```python
from build123d import *

# Parameters (mm, degrees)
SKETCH1_W                      = 133.5
SKETCH1_H                      = 34
BOSS_EXTRUDE1_DEPTH            = 1
SKETCH2_W                      = 10
SKETCH2_H                      = 8.625
BOSS_EXTRUDE2_DEPTH            = 15
SKETCH2_3_W                    = 10
SKETCH2_3_H                    = 16.75
BOSS_EXTRUDE3_DEPTH            = 6.5
CBORE_FOR_M3_SHCS1_D           = 3.4
CBORE_FOR_M3_SHCS1_CBORE_D     = 6.5
CBORE_FOR_M3_SHCS1_CBORE_DEPTH = 3
CHAMFER1_SIZE                  = 0.5
CHAMFER2_SIZE                  = 0.5
CUT_EXTRUDE1_DEPTH             = 71.495123945
LPATTERN1_COUNT                = 3
LPATTERN1_PITCH                = 18.475
MIRROR2_COPY_1_DEPTH           = 71.495123945
MIRROR2_COPY_2_DEPTH           = 71.495123945
MIRROR2_COPY_3_DEPTH           = 71.495123945
CHAMFER3_SIZE                  = 1
INTERSECT1_START               = 14
INTERSECT1_OUTLINE_R           = 1.7
INTERSECT1_DEPTH               = 1


# Read off the part's stored shape, not the designer's step: Intersect1
with BuildPart() as part:
    # Sketch1 → Boss-Extrude1 (new body)
    with BuildSketch(Plane.XY):
        Rectangle(SKETCH1_W, SKETCH1_H)
    extrude(amount=BOSS_EXTRUDE1_DEPTH)

    # Sketch2 → Boss-Extrude2 (add)
    with BuildSketch(Plane.XY):
        with Locations((61.75, -12.6875)):
            Rectangle(SKETCH2_W, SKETCH2_H)
        with Locations((61.75, 12.6875)):
            Rectangle(SKETCH2_W, SKETCH2_H)
    boss_extrude2 = extrude(amount=BOSS_EXTRUDE2_DEPTH)

    # Sketch2<3> → Boss-Extrude3 (add)
    with BuildSketch(Plane.XY):
        with Locations((61.75, 0)):
            Rectangle(SKETCH2_3_W, SKETCH2_3_H)
    boss_extrude3 = extrude(amount=BOSS_EXTRUDE3_DEPTH)

    # CBORE for M3 SHCS1 (through all)
    with Locations(Plane(origin=(0, 0, 0), x_dir=(-1, 0, 0), z_dir=(0, 0, -1))):
        with Locations((-61.75, 12.75), (-61.75, -12.75)):
            cbore_for_m3_shcs1 = CounterBoreHole(CBORE_FOR_M3_SHCS1_D / 2, CBORE_FOR_M3_SHCS1_CBORE_D / 2, CBORE_FOR_M3_SHCS1_CBORE_DEPTH)

    # Chamfer1
    chamfer1_edges = [part.edges().sort_by_distance(p)[0] for p in [
        (61.75, 8.375, 6.5),
        (61.75, -8.375, 6.5),
    ]]
    chamfer(chamfer1_edges, length=CHAMFER1_SIZE)

    # Mirror1: Boss-Extrude2, Boss-Extrude3, CBORE for M3 SHCS1 across plane
    add(boss_extrude2.mirror(Plane(origin=(0, 0, 0), x_dir=(0, 0, 1), z_dir=(1, 0, 0))))
    add(boss_extrude3.mirror(Plane(origin=(0, 0, 0), x_dir=(0, 0, 1), z_dir=(1, 0, 0))))
    add(cbore_for_m3_shcs1.mirror(Plane(origin=(0, 0, 0), x_dir=(0, 0, 1), z_dir=(1, 0, 0))), mode=Mode.SUBTRACT)

    # Chamfer2
    chamfer2_edges = [part.edges().sort_by_distance(p)[0] for p in [
        (-65, -12.75, 0),
        (-65, 12.75, 0),
        (65, -12.75, 0),
        (65, 12.75, 0),
    ]]
    chamfer(chamfer2_edges, length=CHAMFER2_SIZE)

    # Sketch6 → Cut-Extrude1 (cut, through all)
    with BuildSketch(Plane.XY):
        Polygon((-7.505553499, 15), (0, 2), (7.505553499, 15), align=None)
        Polygon((-16.743157806, 1), (-1.732050808, 1), (-9.237604307, 14), align=None)
        Polygon((-16.743157806, -1), (-9.237604307, -14), (-1.732050808, -1), align=None)
        Polygon((1.732050808, 1), (16.743157806, 1), (9.237604307, 14), align=None)
        Polygon((1.732050808, -1), (9.237604307, -14), (16.743157806, -1), align=None)
        Polygon((-7.505553499, -15), (7.505553499, -15), (0, -2), align=None)
    cut_extrude1 = extrude(amount=CUT_EXTRUDE1_DEPTH, mode=Mode.SUBTRACT)

    # LPattern1: Cut-Extrude1 ×3
    with Locations(*[(-i * LPATTERN1_PITCH, 0, 0) for i in range(1, LPATTERN1_COUNT)]):
        add(cut_extrude1, mode=Mode.SUBTRACT)

    # Mirror2 copy 1 sketch → Mirror2 copy 1 (cut, through all)
    with BuildSketch(Plane(origin=(18.475, 0, 0), x_dir=(-1, 0, 0), z_dir=(0, 0, 1))):
        Polygon((-7.505553499, -15), (0, -2), (7.505553499, -15), align=None)
        Polygon((-16.743157806, -1), (-1.732050808, -1), (-9.237604307, -14), align=None)
        Polygon((-16.743157806, 1), (-9.237604307, 14), (-1.732050808, 1), align=None)
        Polygon((1.732050808, -1), (16.743157806, -1), (9.237604307, -14), align=None)
        Polygon((1.732050808, 1), (9.237604307, 14), (16.743157806, 1), align=None)
        Polygon((-7.505553499, 15), (7.505553499, 15), (0, 2), align=None)
    extrude(amount=MIRROR2_COPY_1_DEPTH, mode=Mode.SUBTRACT)

    # Mirror2 copy 2 sketch → Mirror2 copy 2 (cut, through all)
    with BuildSketch(Plane(origin=(36.95, 0, 0), x_dir=(-1, 0, 0), z_dir=(0, 0, 1))):
        Polygon((-7.505553499, -15), (0, -2), (7.505553499, -15), align=None)
        Polygon((-16.743157806, -1), (-1.732050808, -1), (-9.237604307, -14), align=None)
        Polygon((-16.743157806, 1), (-9.237604307, 14), (-1.732050808, 1), align=None)
        Polygon((1.732050808, -1), (16.743157806, -1), (9.237604307, -14), align=None)
        Polygon((1.732050808, 1), (9.237604307, 14), (16.743157806, 1), align=None)
        Polygon((-7.505553499, 15), (7.505553499, 15), (0, 2), align=None)
    extrude(amount=MIRROR2_COPY_2_DEPTH, mode=Mode.SUBTRACT)

    # Mirror2 copy 3 sketch → Mirror2 copy 3 (cut, through all)
    with BuildSketch(Plane(origin=(0, 0, 0), x_dir=(-1, 0, 0), z_dir=(0, 0, 1))):
        Polygon((-7.505553499, -15), (0, -2), (7.505553499, -15), align=None)
        Polygon((-16.743157806, -1), (-1.732050808, -1), (-9.237604307, -14), align=None)
        Polygon((-16.743157806, 1), (-9.237604307, 14), (-1.732050808, 1), align=None)
        Polygon((1.732050808, -1), (16.743157806, -1), (9.237604307, -14), align=None)
        Polygon((1.732050808, 1), (9.237604307, 14), (16.743157806, 1), align=None)
        Polygon((-7.505553499, 15), (7.505553499, 15), (0, 2), align=None)
    extrude(amount=MIRROR2_COPY_3_DEPTH, mode=Mode.SUBTRACT)

    # Chamfer3
    chamfer3_edges = [part.edges().sort_by_distance(p)[0] for p in [
        (66.75, -17, 7.5),
        (-66.75, -17, 7.5),
        (-66.75, 17, 7.5),
        (66.75, 17, 7.5),
    ]]
    chamfer(chamfer3_edges, length=CHAMFER3_SIZE)

    # Intersect1 outline → Intersect1 (cut)
    # profile 1 of 4: a face of its own
    with BuildSketch(Plane.XY.offset(INTERSECT1_START)):
        Polygon((-56.75, 17), (-65.75, 17), (-66.75, 16), (-66.75, 8.375), (-56.75, 8.375), align=None)
        with Locations((-61.75, 12.75)):
            Circle(INTERSECT1_OUTLINE_R, mode=Mode.SUBTRACT)
    # profile 2 of 4: a face of its own
    with BuildSketch(Plane.XY.offset(INTERSECT1_START)):
        Polygon((65.75, 17), (56.75, 17), (56.75, 8.375), (66.75, 8.375), (66.75, 16), align=None)
        with Locations((61.75, 12.75)):
            Circle(INTERSECT1_OUTLINE_R, mode=Mode.SUBTRACT)
    # profile 3 of 4: a face of its own
    with BuildSketch(Plane.XY.offset(INTERSECT1_START)):
        Polygon((-56.75, -17), (-56.75, -8.375), (-66.75, -8.375), (-66.75, -16), (-65.75, -17), align=None)
        with Locations((-61.75, -12.75)):
            Circle(INTERSECT1_OUTLINE_R, mode=Mode.SUBTRACT)
    # profile 4 of 4: a face of its own
    with BuildSketch(Plane.XY.offset(INTERSECT1_START)):
        Polygon((66.75, -8.375), (56.75, -8.375), (56.75, -17), (65.75, -17), (66.75, -16), align=None)
        with Locations((61.75, -12.75)):
            Circle(INTERSECT1_OUTLINE_R, mode=Mode.SUBTRACT)
    extrude(amount=INTERSECT1_DEPTH, mode=Mode.SUBTRACT)


solid = part.part
```
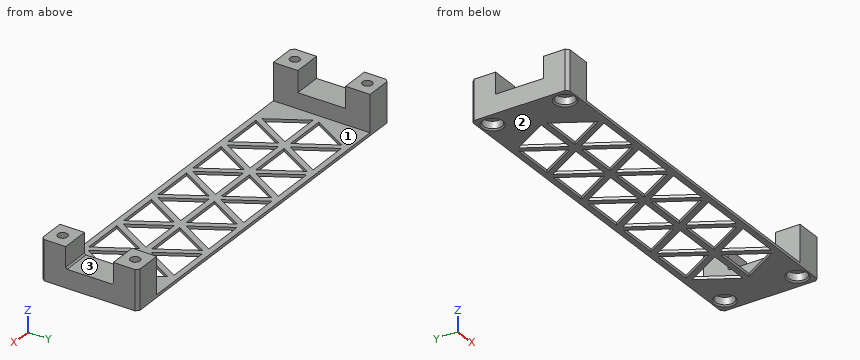
Check sheet for the modelled part. Datum: model origin and axes. Units: mm. Face numbers are marked on the shaded views. A direction names the side the tool comes from. Give positions to 0.01 mm unless a question says otherwise; leave off trailing zeros. Loops run counter-clockwise (first coordinate to the right, second up) from the corner with the lowest first, then second, coordinate; pieces in that order, holes last. Notation, with made-up numbers: M 30,-30.5 L 86,-30.5 A27 cw 86,-5.5 Z; hole C -7.75,-39.75 d6. An arc over 180 degrees is marked long. Answer in a Markdown table with one row per item.
1) Cross-section at B-B (x = -61.75). Enter the section's corners in (y, z) (3 decimals), plus the area to 3 significant figures.
Solutions:
| item | result |
|---|---|
| outline | M -17,0 L -16.5,0 L -16,0.5 L -16,3 L -14.45,3 L -14.45,14 L -17,14 Z; M -11.05,3 L -9.5,3 L -9.5,0.5 L -9,0 L 9,0 L 9.5,0.5 L 9.5,3 L 11.05,3 L 11.05,14 L 8.375,14 L 8.375,6.5 L -8.375,6.5 L -8.375,14 L -11.05,14 Z; M 14.45,3 L 16,3 L 16,0.5 L 16.5,0 L 17,0 L 17,14 L 14.45,14 Z |
| area | 236 mm^2 |
2) Thickness scan on line 1 (Y direction, x = -61.75, z = 1.65); line 2 (Y direction, x = 61.75, z = 9.5) (3 decimals); line 3 (X direction, y = 3, z = 4). Record the ranges inside material, lowest first.
Solutions:
| item | result |
|---|---|
| line 1 | y = -17 to -16, -9.5 to 9.5, 16 to 17 |
| line 2 | y = -17 to -14.45, -11.05 to -8.375, 8.375 to 11.05, 14.45 to 17 |
| line 3 | x = -66.75 to -56.75, 56.75 to 66.75 |
3) Cross-section at C-C (x = -4). Enter the section's corners in (y, z).
Solutions:
| item | result |
|---|---|
| outline | M -17,0 L -15,0 L -15,1 L -17,1 Z; M -8.93,0 L -4.93,0 L -4.93,1 L -8.93,1 Z; M -1,0 L 1,0 L 1,1 L -1,1 Z; M 4.93,0 L 8.93,0 L 8.93,1 L 4.93,1 Z; M 15,0 L 17,0 L 17,1 L 15,1 Z |
4) Tool access check on the marked faces 1, 2 and 3. Record the directions out of +Z, -Z, +X, -X, +Y, -Y that give a thin tool (end or side, any length) a straight path to the whole face; none if there is none.
Solutions:
| item | result |
|---|---|
| face 1 | +Z, +Y, -Y |
| face 2 | -Z, +X, -X, +Y, -Y |
| face 3 | +Z, +X, -X |
5) Depth check by flat-ended pin: pin 1 (3 mm diameter, centred on x = 61.5, y = 11.5, fed in from -Z); pin 2 (5 mm diameter, centred on x = 32, y = -7, fed in from +Z); pin 3 (3 mm diameter, centred on x = -63.5, y = 2, fed in from +Z). Enter the tip coordinate at first touch or a pass-through.
Solutions:
| item | result |
|---|---|
| pin 1 | stops at z = 3 |
| pin 2 | stops at z = 1 |
| pin 3 | stops at z = 6.5 |
6) Cross-section at D-D (x = 61.75). Count the separate pieces of the cut face and the enclosed holes in it, plus the area to 3 significant figures.
Solutions:
| item | result |
|---|---|
| separate pieces | 3 |
| enclosed holes | 0 |
| area | 236 mm^2 |
7) Cross-section at A-A (z = 9.25). Enter the section's corners in (x, y) (3 decimals), plus the area to 3 significant figures.
Solutions:
| item | result |
|---|---|
| outline | M -66.75,-16 L -65.75,-17 L -56.75,-17 L -56.75,-8.375 L -66.75,-8.375 Z; M -66.75,8.375 L -56.75,8.375 L -56.75,17 L -65.75,17 L -66.75,16 Z; M 56.75,-17 L 65.75,-17 L 66.75,-16 L 66.75,-8.375 L 56.75,-8.375 Z; M 56.75,8.375 L 66.75,8.375 L 66.75,16 L 65.75,17 L 56.75,17 Z; hole C -61.75,-12.75 d3.4; hole C -61.75,12.75 d3.4; hole C 61.75,-12.75 d3.4; hole C 61.75,12.75 d3.4 |
| area | 307 mm^2 |
